The model under review builds one solid part; all positions refer to its coordinate system, in mm. A direction names the side the tool comes from. Round coordinates to 2 decimals unless told otherwise and drop trailing zeros. Loops run counter-clockwise (first coordinate to the right, second up) from the corner with the lowest first, then second, coordinate; pieces in that order, holes last. Notation, with made-up numbers: M 22.5,42 L 43.5,42 A8 ccw 43.5,49 Z; hole C 4.25,15.5 d7. An arc over 180 degrees is marked long. One line per question, with ' | ' between items.
from build123d import *

# Parameters (mm, degrees)
F0_W      = 45
F0_H      = 45
F1_DEPTH  = 2795
F3_W      = 90
F3_H      = 60
F4_DEPTH  = 5
F6_DEPTH  = 45
F8_W      = 2.7798460424
F8_H      = 5.7082939148
F9_DEPTH  = 150
F10_R     = 6
F11_DEPTH = 5
F15_DEPTH = 30


with BuildPart() as f1:
    # F0 (on Top) → F1 (new body)
    with BuildSketch(Plane.XY):
        Rectangle(F0_W, F0_H)
    extrude(amount=F1_DEPTH)


with BuildPart() as f4:
    # F3 (on face) → F4 (new body)
    with BuildSketch(Plane(origin=(0, -524.3318959349, 2697.453760933), x_dir=(1, 0, 0), z_dir=(0, -0.1908089954, 0.9816271834))):
        Polygon((-22.5, 661.2245304499), (-22.5, 511.2245304499), (37.5, 511.2245304499), (37.5, 571.2245304499), (37.5, 661.2245304499), align=None)
        with Locations((82.5, 541.2245304499)):
            Rectangle(F3_W, F3_H)
    extrude(amount=F4_DEPTH)


with BuildPart() as f6:
    # F5 (on face) → F6 (new body)
    with BuildSketch(Plane.YZ.offset(22.5)):
        Polygon((-22.5, 2795), (22.5, 2795), (22.5, 2803.7471139112), align=None)
    extrude(amount=-F6_DEPTH)


with BuildPart() as f1_1:
    add(f1.part)

    # F7: union F6, F4
    add(f6.part)
    add(f4.part)

    # F8 (on face) → F9 (cut, through all)
    with BuildSketch(Plane(origin=(-22.5, 0, 0), x_dir=(0, -1, 0), z_dir=(-1, 0, 0))):
        with Locations((23.8899230212, 2797.8541469574)):
            Rectangle(F8_W, F8_H)
    extrude(amount=-F9_DEPTH, mode=Mode.SUBTRACT)

    # F10 (on face) → F11 (cut, through all)
    with BuildSketch(Plane(origin=(0, -525.2859409117, 2702.3618968503), x_dir=(1, 0, 0), z_dir=(0, -0.1908089954, 0.9816271834))):
        with BuildLine():
            ThreePointArc((108.5, 556.2245304499), (106.7426406871, 560.467171137), (102.5, 562.2245304499))
            Line((102.5, 562.2245304499), (102.5, 556.2245304499))
            Line((102.5, 556.2245304499), (96.5, 556.2245304499))
            ThreePointArc((96.5, 556.2245304499), (102.5, 550.2245304499), (108.5, 556.2245304499))
        make_face()
        with Locations((62.5, 556.2245304499)):
            Circle(F10_R)
        with BuildLine():
            Line((102.5, 556.2245304499), (102.5, 562.2245304499))
            ThreePointArc((102.5, 562.2245304499), (98.2573593129, 560.467171137), (96.5, 556.2245304499))
            Line((96.5, 556.2245304499), (102.5, 556.2245304499))
        make_face()
        with BuildLine():
            ThreePointArc((22.5, 630.2245304499), (26.7426406871, 631.9818897628), (28.5, 636.2245304499))
            Line((28.5, 636.2245304499), (22.5, 636.2245304499))
            Line((22.5, 636.2245304499), (22.5, 630.2245304499))
        make_face()
        with BuildLine():
            Line((22.5, 636.2245304499), (28.5, 636.2245304499))
            ThreePointArc((28.5, 636.2245304499), (18.2573593129, 640.467171137), (22.5, 630.2245304499))
            Line((22.5, 630.2245304499), (22.5, 636.2245304499))
        make_face()
        with BuildLine():
            ThreePointArc((28.5, 596.2245304499), (26.7426406871, 600.467171137), (22.5, 602.2245304499))
            ThreePointArc((22.5, 602.2245304499), (18.2573593129, 591.9818897628), (28.5, 596.2245304499))
        make_face()
    extrude(amount=-F11_DEPTH, mode=Mode.SUBTRACT)

    # F13 (on offset) → F15 (join)
    with BuildSketch(Plane.XY.offset(2545)):
        with BuildLine():
            ThreePointArc((-5, 27.5), (-3.5355339059, 23.9644660941), (0, 22.5))
            Line((0, 22.5), (0, 27.5))
            Line((0, 27.5), (-5, 27.5))
        make_face()
        with BuildLine():
            Line((-5, 22.5), (0, 22.5))
            ThreePointArc((0, 22.5), (-3.5355339059, 23.9644660941), (-5, 27.5))
            Line((-5, 27.5), (-5, 22.5))
        make_face()
        with BuildLine():
            Line((0, 27.5), (0, 22.5))
            ThreePointArc((0, 22.5), (3.5355339059, 23.9644660941), (5, 27.5))
            Line((5, 27.5), (0, 27.5))
        make_face()
        with BuildLine():
            ThreePointArc((5, 27.5), (3.5355339059, 23.9644660941), (0, 22.5))
            Line((0, 22.5), (5, 22.5))
            Line((5, 22.5), (5, 27.5))
        make_face()
        with BuildLine():
            Line((-5, 27.5), (0, 27.5))
            Line((0, 27.5), (5, 27.5))
            ThreePointArc((5, 27.5), (0, 32.5), (-5, 27.5))
        make_face()
    extrude(amount=F15_DEPTH)

    # F17: sweep along a path in F14
    with BuildLine(Plane.YZ) as f17_path:
        ThreePointArc((57.5, 2575), (42.5, 2590), (27.5, 2575))
    # F16 (on face) → F17 (sweep)
    with BuildSketch(Plane.XY.offset(2575)):
        with BuildLine():
            ThreePointArc((0, 22.5), (3.5355339059, 23.9644660941), (5, 27.5))
            ThreePointArc((5, 27.5), (0, 32.5), (-5, 27.5))
            ThreePointArc((-5, 27.5), (-3.5355339059, 23.9644660941), (0, 22.5))
        make_face()
    sweep(path=f17_path.line)


solid = f1_1.part
1) Add section A-A on z = 1995. State the section outline as (x, y) points, then the cut area to 4 significant figures.
Output values:
outline: M -22.5,-22.5 L 22.5,-22.5 L 22.5,22.5 L -22.5,22.5 Z | area: 2,025 mm²
2) Machinability: for faces 1 (the flat face through (22.5, 0, 1421)), 2 (the flat face through (0, 0, 0)), which of the approach directions +Z, -Z, +X, -X, +Y, -Y give a long, thin tool a straight path to every point of the face, cutting with its end or side? Answer none if there is none.
Output values:
face 1: -Z, +X, +Y, -Y | face 2: -Z, +X, -X, +Y, -Y
3) For line 1 (X direction, y = -7.5, z = 1973); line 2 (Z direction, x = -9, y = 23.5), list the stretches that pass through material, from the lowest coordinate up.
Output values:
line 1: x = -22.5 to 22.5 | line 2: z = 2803.94 to 2809.04
4) Insertion check: P1, Ø5, axis at x = 34, y = 77.5, coming from the +Z side; P2, Ø10, axis at y = -7, z = 472.5, coming from the +X side; P3, Ø6, axis at x = -5, z = 834.5, coming from the +Y side. Each pin has a flat end and moves straight along its axis. Give the tip position at first contact, or say it passes through.
Output values:
P1: stops at z = 2820.02 | P2: stops at x = 22.5 | P3: stops at y = 22.5
